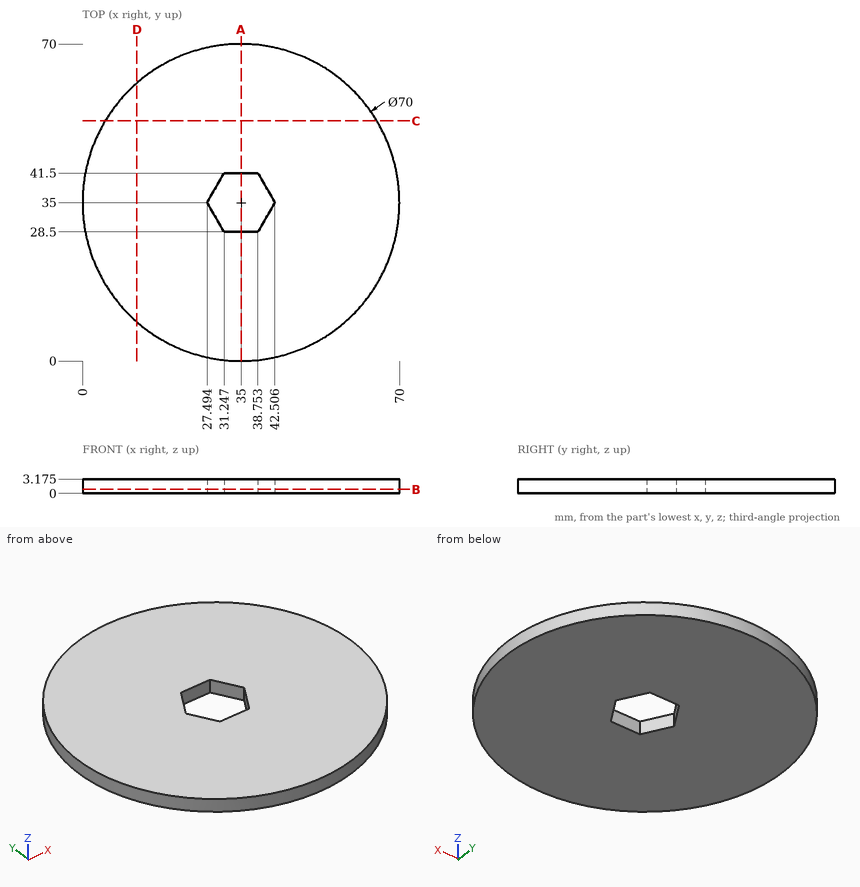
Design review of the part shown in the three views and the two pictorial views. Dimensions are in mm from the part's minimum x, y and z. Give positions to 0.01 mm unless a question says otherwise; leave off trailing zeros. Loops run counter-clockwise (first coordinate to the right, second up) from the corner with the lowest first, then second, coordinate; pieces in that order, holes last. Notation, with made-up numbers: (-34, -34) -> (16, -34) arc R19 cw to (16, -29) -> close; hole circle Ø8 at (41.25, 76). An arc over 180 degrees is marked (long way). Answer as a JSON object with one key per item and string values. Group by question number.
Q1. Take a section at B-B (z = 0.9). Write out the cut boundary in (x, y) (1 decimal).
Q2. Insertion check: pin 1 (1 mm diameter, centred on y = 47, z = 0.5, fed in from -X). The pin has a flat end and moves straight along its axis. Give the tip position at first contact, or say it passes through.
Q3. Take a section at C-C (y = 53). Write out the cut boundary in (x, z) (1 decimal).
Q4. Take a section at D-D (x = 12). Write out the cut boundary in (y, z) (1 decimal).
Q5. Take a section at A-A (x = 35). Write out the cut boundary in (y, z) (1 decimal).
Q6. Wall thickness on line 1 along Y through (x, z) = (29, 1.2) (1 decimal); line 2 along Y through (x, z) = (35, 1.55); line 3 along Y through (x, z) = (16.5, 2.85): over which ranges is each line inside the solid? List them lowest first.
Answer below:
{
 "1": {"outline": "circle Ø70 at (35, 35); hole (27.5, 35) -> (31.2, 28.5) -> (38.8, 28.5) -> (42.5, 35) -> (38.8, 41.5) -> (31.2, 41.5) -> close"},
 "2": {"pin 1": "stops at x = 1.94"},
 "3": {"outline": "(5, 0) -> (65, 0) -> (65, 3.2) -> (5, 3.2) -> close"},
 "4": {"outline": "(8.6, 0) -> (61.4, 0) -> (61.4, 3.2) -> (8.6, 3.2) -> close"},
 "5": {"outline": "(0, 0) -> (28.5, 0) -> (28.5, 3.2) -> (0, 3.2) -> close; (41.5, 0) -> (70, 0) -> (70, 3.2) -> (41.5, 3.2) -> close"},
 "6": {"line 1": "y = 0.5 to 32.4, 37.6 to 69.5", "line 2": "y = 0 to 28.5, 41.5 to 70", "line 3": "y = 5.29 to 64.71"}
}
